Can you work these out from the drawing? Everything is in mm from the part's minimum corner. A direction names the side the tool comes from. Coordinates: 2 decimals unless noted, no trailing zeros. Order: outer loops, then holes, each group sorted by start corner. A loop starts at its lowest first (then second) coordinate and runs counter-clockwise, first axis right, second up. Notation, with made-up numbers: (-40, 18.25) -> (-26, 18.25) arc R20 ccw to (-26, 38.25) -> close; hole circle Ø2 at (71.5, 49.5). An arc over 180 degrees is marked (long way). Answer in a Markdown table with one row per item.
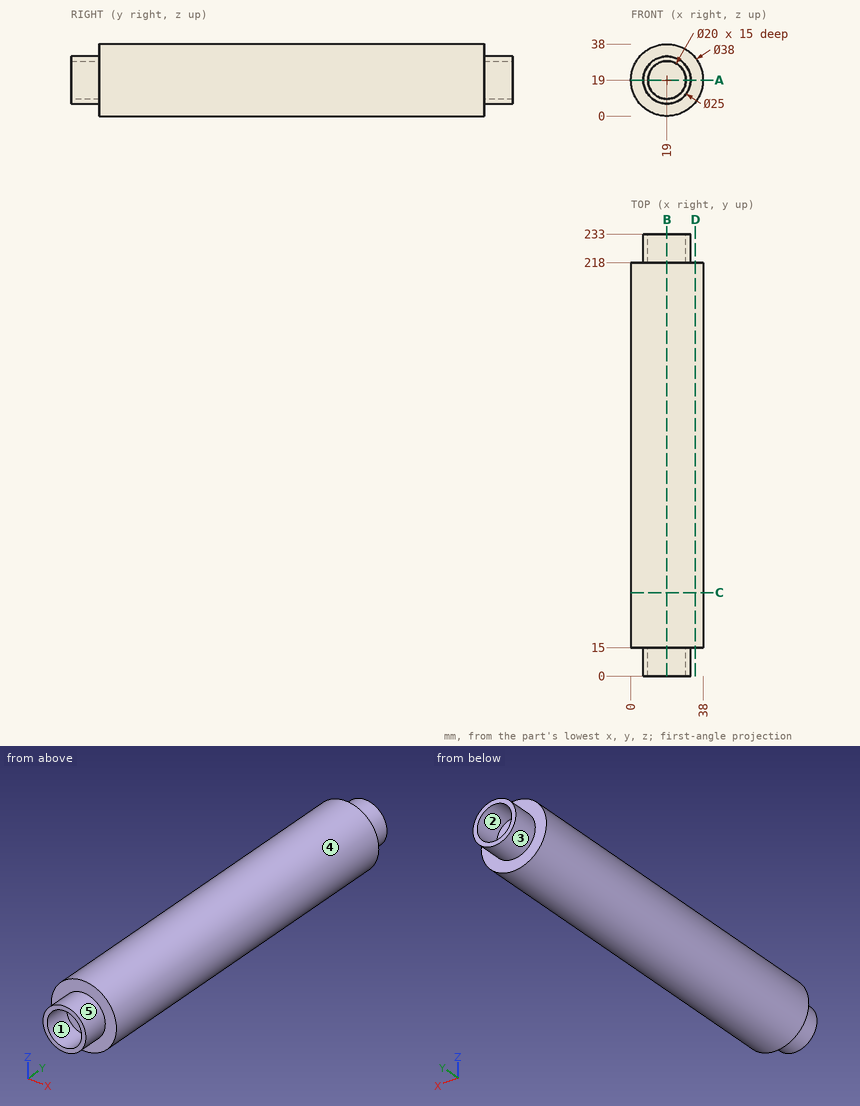
(1) Suppose I cut it at A-A (z = 19). Please give me the cut outline in (x, y).
Response values:
| item | result |
|---|---|
| outline | (0, 15) -> (6.5, 15) -> (6.5, 0) -> (9, 0) -> (9, 15) -> (29, 15) -> (29, 0) -> (31.5, 0) -> (31.5, 15) -> (38, 15) -> (38, 218) -> (31.5, 218) -> (31.5, 233) -> (29, 233) -> (29, 218) -> (9, 218) -> (9, 233) -> (6.5, 233) -> (6.5, 218) -> (0, 218) -> close |
(2) Suppose I cut it at B-B (x = 19). Please give me the cut outline in (y, z).
Response values:
| item | result |
|---|---|
| outline | (0, 6.5) -> (15, 6.5) -> (15, 0) -> (218, 0) -> (218, 6.5) -> (233, 6.5) -> (233, 9) -> (218, 9) -> (218, 29) -> (233, 29) -> (233, 31.5) -> (218, 31.5) -> (218, 38) -> (15, 38) -> (15, 31.5) -> (0, 31.5) -> (0, 29) -> (15, 29) -> (15, 9) -> (0, 9) -> close |
(3) On a 3-axis mill with a long thin cutter (end or side, diameter ignored), from which of +Z, -Z, +X, -X, +Y, -Y can I reach the whole of each face in a straight line? I mean the marked faces 4 and 5. Say none if no direction works.
Response values:
| item | result |
|---|---|
| face 4 | +Y, -Y |
| face 5 | -Y |
(4) I need wall thicknesses on line 1 (X direction, y = 8, z = 19); line 2 (Y direction, x = 25.5, z = 6.5); line 3 (Z direction, x = 17, y = 13.5). Which ranges of each line are inside material? Lowest first, please. Write a range as [from, to].
Response values:
| item | result |
|---|---|
| line 1 | [6.5, 9], [29, 31.5] |
| line 2 | [15, 218] |
| line 3 | [6.66, 9.2], [28.8, 31.34] |
(5) We'd pull the mould along X, two halves only. Please class the marked faces 1, 2 and 3: +X half, -X half, draft (parallel to the pull), parting line (faces both ways), or undercut.
Response values:
| item | result |
|---|---|
| face 1 | undercut |
| face 2 | undercut |
| face 3 | parting line |
(6) Will these pins go through, and if not, where does the flat tip stop? pin 1 Ø10 at (x, y) = (30.5, 32.5) entering from +Z; pin 2 Ø6 at (x, z) = (31.5, 30) entering from +Y; pin 3 Ø16 at (x, z) = (14.5, 15) entering from -Y; pin 4 Ø1.5 at (x, y) = (4, 25.5) entering from +Z.
Response values:
| item | result |
|---|---|
| pin 1 | z = 36.85 |
| pin 2 | y = 218 |
| pin 3 | y = 0 |
| pin 4 | z = 31.57 |
(7) Suppose I cut it at D-D (x = 34). Please give me the cut outline in (y, z), and give its area (3 significant figures).
Response values:
| item | result |
|---|---|
| outline | (15, 7.34) -> (218, 7.34) -> (218, 30.66) -> (15, 30.66) -> close |
| area | 4,730 mm2 |
(8) Suppose I cut it at C-C (y = 44). Please give me the cut outline in (x, z).
Response values:
| item | result |
|---|---|
| outline | circle Ø38 at (19, 19) |
